```python
from build123d import *

# Parameters (mm, degrees)
BOSS_EXTRUDE1_DEPTH      = 30
BOSS_EXTRUDE1_DEPTH_BACK = 30
SKETCH1_R                = 3
SKETCH2_R                = 3.5
BOSS_EXTRUDE2_DEPTH      = 1
BOSS_EXTRUDE3_START      = 1
SKETCH3_R                = 3.5
BOSS_EXTRUDE3_DEPTH      = 1


with BuildPart() as part:
    # Sketch1 → Boss-Extrude1 (new, two sides: drawn at the far end of the back side and taken through both)
    with BuildSketch(Plane.XY.offset(-BOSS_EXTRUDE1_DEPTH_BACK)):
        Circle(SKETCH1_R)
    extrude(amount=BOSS_EXTRUDE1_DEPTH + BOSS_EXTRUDE1_DEPTH_BACK)

    # Sketch2 → Boss-Extrude2 (add)
    with BuildSketch(Plane.XY.offset(30)):
        Circle(SKETCH2_R)
    extrude(amount=BOSS_EXTRUDE2_DEPTH)

    # Sketch3 → Boss-Extrude3 (add)
    with BuildSketch(Plane(origin=(0, 0, -30), x_dir=(-1, 0, 0), z_dir=(0, 0, -1)).offset(BOSS_EXTRUDE3_START)):
        with Locations(Location((0, 0, 0), (0, 0, 180))):
            Circle(SKETCH3_R)
    extrude(amount=-BOSS_EXTRUDE3_DEPTH)


solid = part.part
```
Geometry check sheet. Reference: the model listing, model coordinates, mm. A direction names the side the tool comes from. Give positions to 0.01 mm unless a question says otherwise; leave off trailing zeros. Order: outer loops, then holes, each group sorted by start corner. A loop starts at its lowest first (then second) coordinate and runs counter-clockwise, first axis right, second up.
1. Access from +Z, -Z, +X, -X, +Y, -Y to the whole of each face (thin tool, end or side, straight path). Record for faces 4 (the face through (0, 0, -31)), 5 (the face through (3, 1, 30)).
2. Section check C-C, the plane z = -7. Enter the section's corners in (x, y).
3. Section check A-A, the plane x = 0. Enter the section's corners in (y, z), and give its area (3 significant figures).
4. Release check for a two-part mould opening along Z. For faces 1 (the face through (-3, 0, 0)), 2 (the face through (0, 0, 31)), 3 (the face through (3.233, -1.341, 30.493)) record: pulls with the +Z half, pulls with the -Z half, needs draft (parallel to the pull), parting line crosses it, or undercut.
5. Gauge pin test, flat end, axial feed: pin 1 Ø1.5 at (y, z) = (-0.5, -11) entering from +X. Record the tip position at first contact, or that the pin passes through.
6. Thickness scan on L1, parallel to Y at x = -0.25, z = 18.5; L2, parallel to X at y = 0.75, z = 16.5. Record the ranges inside material, lowest first.
Values follow:
1. face 4: -Z, +X, -X, +Y, -Y
1. face 5: none
2. outline: circle Ø6 at (0, 0)
3. outline: (-3.5, -31) - (3.5, -31) - (3.5, -30) - (3, -30) - (3, 30) - (3.5, 30) - (3.5, 31) - (-3.5, 31) - (-3.5, 30) - (-3, 30) - (-3, -30) - (-3.5, -30) - close
3. area: 374 mm2
4. face 1: undercut
4. face 2: pulls with the +Z half
4. face 3: needs draft
5. pin 1: stops at x = 3
6. L1: y = -2.99 to 2.99
6. L2: x = -2.9 to 2.9
